from build123d import *

# Parameters (mm, degrees)
SHEET_EXTRUDE_1_1_DEPTH = 50
THICKEN_1_T1            = 2
SHEET_METAL_1_DEPTH     = 50
SHEET_METAL_1_2_DEPTH   = 50


# Read off the part's stored shape, not the designer's step: Преобразовать-Твердое тело1
with BuildPart() as body_1:
    # Sheet Extrude 1: a surface, the sketch's curves swept straight by 50 mm
    with BuildLine(Plane.XY, mode=Mode.PRIVATE) as sheet_extrude_1_1_path:
        Line((-55.428908385, 46.043182684), (61.804118295, 46.043182684))
        Line((61.804118295, 46.043182684), (61.804118295, -50.293322624))
        Line((61.804118295, -50.293322624), (-55.428908385, -50.293322624))
        Line((-55.428908385, -50.293322624), (-55.428908385, 46.043182684))
    sheet_extrude_1_1 = Shell.extrude(sheet_extrude_1_1_path.wire(), (0 * SHEET_EXTRUDE_1_1_DEPTH, 0 * SHEET_EXTRUDE_1_1_DEPTH, 1 * SHEET_EXTRUDE_1_1_DEPTH))
    add(Solid.thicken(sheet_extrude_1_1, THICKEN_1_T1))

    # Sheet Metal 1 outline → Sheet Metal 1 (cut)
    with BuildSketch(Plane.XY):
        Polygon((61.804118295, 46.043182684), (61.804118295, 42.628969122), (63.804118295, 42.628969122), (63.804118295, 48.043182684), (58.389904733, 48.043182684), (58.389904733, 46.043182684), align=None)
        with BuildLine():
            Line((63.804118295, -52.293322624), (63.804118295, -49.293322624))
            ThreePointArc((63.804118295, -49.293322624), (62.925438639, -51.414642968), (60.804118295, -52.293322624))
            Line((60.804118295, -52.293322624), (63.804118295, -52.293322624))
        make_face()
        with BuildLine():
            Line((-57.428908385, -52.293322624), (-54.428908385, -52.293322624))
            ThreePointArc((-54.428908385, -52.293322624), (-56.550228729, -51.414642968), (-57.428908385, -49.293322624))
            Line((-57.428908385, -49.293322624), (-57.428908385, -52.293322624))
        make_face()
        with BuildLine():
            ThreePointArc((-57.428908385, 45.043182684), (-56.550228729, 47.164503028), (-54.428908385, 48.043182684))
            Line((-54.428908385, 48.043182684), (-57.428908385, 48.043182684))
            Line((-57.428908385, 48.043182684), (-57.428908385, 45.043182684))
        make_face()
    extrude(amount=SHEET_METAL_1_DEPTH, mode=Mode.SUBTRACT)

    # Sheet Metal 1 2 outline → Sheet Metal 1 2 (add)
    with BuildSketch(Plane.XY):
        with BuildLine():
            Line((61.804118295, -50.293322624), (61.804118295, -49.293322624))
            ThreePointArc((61.804118295, -49.293322624), (61.511225076, -50.000429405), (60.804118295, -50.293322624))
            Line((60.804118295, -50.293322624), (61.804118295, -50.293322624))
        make_face()
        with BuildLine():
            Line((-55.428908385, -50.293322624), (-54.428908385, -50.293322624))
            ThreePointArc((-54.428908385, -50.293322624), (-55.136015166, -50.000429405), (-55.428908385, -49.293322624))
            Line((-55.428908385, -49.293322624), (-55.428908385, -50.293322624))
        make_face()
        with BuildLine():
            ThreePointArc((-55.428908385, 45.043182684), (-55.136015166, 45.750289465), (-54.428908385, 46.043182684))
            Line((-54.428908385, 46.043182684), (-55.428908385, 46.043182684))
            Line((-55.428908385, 46.043182684), (-55.428908385, 45.043182684))
        make_face()
    extrude(amount=SHEET_METAL_1_2_DEPTH)


solid = body_1.part
Could you check a few things on this model? Use its own coordinates, in mm. A direction names the side the tool comes from. Give positions to 0.01 mm unless a question says otherwise; leave off trailing zeros. Order: outer loops, then holes, each group sorted by start corner. A loop starts at its lowest first (then second) coordinate and runs counter-clockwise, first axis right, second up. Notation, with made-up numbers: (-22.75, 55) - (25.25, 55) arc R18 cw to (25.25, 87) - close; hole circle Ø2 at (-27, -36.75). An arc over 180 degrees is marked (long way). Return JSON: item names as keys, results as strings. Group by question number.
Q1. Suppose I cut it at A-A, the plane x = -21. Please give me the cut outline in (y, z), and give its area (3 significant figures).
Q2. Please list where these lines run through material, in increasing order: line 1 along X through (y, z) = (37.5, 21); line 2 along Y through (x, z) = (48, 8.5). Write a range as [from, to].
Q3. Will these pins go through, and if not, where does the flat tip stop? pin 1 Ø1.6 at (x, z) = (62.5, 14.5) entering from +Y; pin 2 Ø0.6 at (y, z) = (47, 30) entering from +X.
Q4. Suppose I cut it at B-B, the plane y = 37. Please give me the cut outline in (x, z), and give its area (3 significant figures).
Q5. Thinking about a two-plate mould opening in Y: for faces 1 (the face through (-56.527, -51.438, 24.65)), 2 (the face through (-56.573, 47.141, 24.65)), 3 (the face through (61.804, -3, 25)), 4 (the face through (1, 46.043, 25)), which applies, pulls with the +Y half, pulls with the -Y half, needs draft (parallel to the pull), parting line crosses it, or undercut?
Q6. Suppose I cut it at C-C, the plane z = 3. Please give me the cut outline in (x, y).
Q7. Which directions (+Z, -Z, +X, -X, +Y, -Y) give clear straight access to the entire face, cutting with the end or side of a thin tool? Please do faces 5 (the face through (4, -52.293, 25)), 6 (the face through (4, -50.293, 25)).
Resolved:
{
 "1": {"outline": "(-52.29, 0) - (-50.29, 0) - (-50.29, 50) - (-52.29, 50) - close; (46.04, 0) - (48.04, 0) - (48.04, 50) - (46.04, 50) - close", "area": "200 mm2"},
 "2": {"line 1": "x = [-57.43, -55.43], [61.8, 63.8]", "line 2": "y = [-52.29, -50.29], [46.04, 48.04]"},
 "3": {"pin 1": "stops at y = 42.63", "pin 2": "stops at x = 58.39"},
 "4": {"outline": "(-57.43, 0) - (-55.43, 0) - (-55.43, 50) - (-57.43, 50) - close; (61.8, 0) - (63.8, 0) - (63.8, 50) - (61.8, 50) - close", "area": "200 mm2"},
 "5": {"face 1": "pulls with the -Y half", "face 2": "pulls with the +Y half", "face 3": "needs draft", "face 4": "undercut"},
 "6": {"outline": "(-57.43, -49.29) arc R3 ccw to (-54.43, -52.29) - (60.8, -52.29) arc R3 ccw to (63.8, -49.29) - (63.8, 42.63) - (61.8, 42.63) - (61.8, -49.29) arc R1 cw to (60.8, -50.29) - (-54.43, -50.29) arc R1 cw to (-55.43, -49.29) - (-55.43, 45.04) arc R1 cw to (-54.43, 46.04) - (58.39, 46.04) - (58.39, 48.04) - (-54.43, 48.04) arc R3 ccw to (-57.43, 45.04) - close"},
 "7": {"face 5": "+Z, -Z, +X, -X, -Y", "face 6": "+Z, -Z"}
}
